Verification items for the finished model (mm, model axes). A direction names the side the tool comes from. Give positions to 0.01 mm unless a question says otherwise; leave off trailing zeros. Loops run counter-clockwise (first coordinate to the right, second up) from the corner with the lowest first, then second, coordinate; pieces in that order, holes last. Notation, with made-up numbers: (6.5, -5.75) - (56.5, -5.75) arc R15 cw to (56.5, 14.25) - close; hole circle Ø8 at (-12.5, 75.25). An arc over 180 degrees is marked (long way). One line per item, written item: value. Start each with the question number.
1. Sectioned sample at B-B (x = -25). Record the cut outline in (y, z).
2. Gauge pin test, flat ends, axial feed: pin 1 (12.5 mm diameter, centred on x = -67, y = 50, fed in from +Z); pin 2 (1 mm diameter, centred on y = 3.5, z = 1.5, fed in from -X); pin 3 (4 mm diameter, centred on x = 52, z = -4.5, fed in from -Y); pin 4 (0.6 mm diameter, centred on x = -48, z = 0.5, fed in from +Y). Record the tip position at first contact, or that the pin passes through.
3. Scan lines: L1, parallel to Y at x = 37.5, z = 1.75; L2, parallel to X at y = 13, z = -14.25; L3, parallel to Z at x = -49, y = 149. Record each from-to range of solid material in increasing order. Write a range as [from, to].
4. Sectioned sample at A-A (z = -4). Record the cut outline in (x, y).
5. Sectioned sample at D-D (x = 78). Record the cut outline in (y, z).
6. Access from +Z, -Z, +X, -X, +Y, -Y to the whole of each face (thin tool, end or side, straight path). Record for faces 1 (the flat face through (94.815, 76, -10)), 2 (the flat face through (0, 17, 2)), 3 (the flat face through (75, 40, 0)), 4 (the flat face through (-77, 40, 0)).
7. Mould release check, pull along Y, two halves, no side actions. Record for faces 5 (the flat face through (1, 0, 1)), 6 (the flat face through (54.815, 74, -10)), 7 (the flat face through (-76, 110, 0)): pulls with the +Y half, pulls with the -Y half, needs draft (parallel to the pull), parting line crosses it, or undercut.
8. Sectioned sample at C-C (y = 67). Record the cut outline in (x, z).
from build123d import *

# Parameters (mm, degrees)
F1_DEPTH = 2
F3_DEPTH = 2
F4_DEPTH = 3
F5_DEPTH = 2
F6_W     = 40
F6_H     = 10
F6_H_2   = 60
F7_DEPTH = 20


with BuildPart() as f1:
    # F0 (on Top) → F1 (new body)
    with BuildSketch(Plane.XY):
        Polygon((-12.130910923, 0), (0, 0), (12.130910923, 0), (12.130910923, 200), (-12.130910923, 200), align=None)
    extrude(amount=F1_DEPTH)

    # F2 (on Top) → F3 (join)
    with BuildSketch(Plane.XY):
        Polygon((-97.5, 0), (0, 0), (97.5, 0), (97.5, 10), (-97.5, 10), align=None)
        Polygon((-97.5, 70), (0, 70), (97.5, 70), (97.5, 80), (-97.8855118155, 80), align=None)
        Polygon((-97.8855118155, 140), (0, 140), (97.5, 140), (97.5, 150), (-97.8855118155, 150), align=None)
    extrude(amount=F3_DEPTH)

    # F2 (on Top) → F4 (join)
    with BuildSketch(Plane.XY):
        Polygon((-97.5, 70), (0, 70), (97.5, 70), (97.5, 80), (-97.8855118155, 80), align=None)
        Polygon((-97.8855118155, 140), (0, 140), (97.5, 140), (97.5, 150), (-97.8855118155, 150), align=None)
    extrude(amount=F4_DEPTH)

    # F2 (on Top) → F5 (join)
    with BuildSketch(Plane.XY):
        Polygon((-97.5, 0), (0, 0), (97.5, 0), (97.5, 10), (-97.5, 10), align=None)
        Polygon((-97.5, 70), (0, 70), (97.5, 70), (97.5, 80), (-97.8855118155, 80), align=None)
        Polygon((-97.8855118155, 140), (0, 140), (97.5, 140), (97.5, 150), (-97.8855118155, 150), align=None)
    extrude(amount=F5_DEPTH)

    # F6 (on face) → F7 (join)
    with BuildSketch(Plane(origin=(0, 0, 0), x_dir=(1, 0, 0), z_dir=(0, 0, -1))):
        Polygon((-57.4945055695, 0), (-97.5, 0), (-97.3342470533, -10), (-57.3287526228, -10), align=None)
        Polygon((-57.3287526228, -10), (-97.3342470533, -10), (-96.3397293732, -70), (-56.3342349427, -70), align=None)
        with Locations((74.8154554615, -5)):
            Rectangle(F6_W, F6_H)
        Polygon((-56.3342349427, -70), (-96.3397293732, -70), (-96.1739764266, -80), (-56.168481996, -80), align=None)
        with Locations((74.8154554615, -40)):
            Rectangle(F6_W, F6_H_2)
        Polygon((-56.168481996, -80), (-96.1739764266, -80), (-95.1794587465, -140), (-55.173964316, -140), align=None)
        with Locations((74.8154554615, -75)):
            Rectangle(F6_W, F6_H)
        Polygon((-55.173964316, -140), (-95.1794587465, -140), (-95.0137057998, -150), (-55.0082113693, -150), align=None)
        with Locations((74.8154554615, -110)):
            Rectangle(F6_W, F6_H_2)
        with Locations((74.8154554615, -145)):
            Rectangle(F6_W, F6_H)
    extrude(amount=F7_DEPTH)


solid = f1.part
Results are:
1. outline: (0, 0) - (10, 0) - (10, 2) - (0, 2) - close; (70, 0) - (80, 0) - (80, 3) - (70, 3) - close; (140, 0) - (150, 0) - (150, 3) - (140, 3) - close
2. pin 1: stops at z = 0
2. pin 2: stops at x = -97.5
2. pin 3: passes through
2. pin 4: stops at y = 150
3. L1: y = [0, 10], [70, 80], [140, 150]
3. L2: x = [-97.28, -57.28], [54.82, 94.82]
3. L3: z = [0, 3]
4. outline: (-97.5, 0) - (-57.49, 0) - (-55.01, 150) - (-95.01, 150) - close; (54.82, 0) - (94.82, 0) - (94.82, 150) - (54.82, 150) - close
5. outline: (0, -20) - (150, -20) - (150, 3) - (140, 3) - (140, 0) - (80, 0) - (80, 3) - (70, 3) - (70, 0) - (10, 0) - (10, 2) - (0, 2) - close
6. face 1: -Z, +X, +Y, -Y
6. face 2: +Z, +X, -X, -Y
6. face 3: +Z, +X
6. face 4: +Z, -X
7. face 5: pulls with the -Y half
7. face 6: needs draft
7. face 7: undercut
8. outline: (-96.39, -20) - (-56.38, -20) - (-56.38, 0) - (-96.39, 0) - close; (-12.13, 0) - (12.13, 0) - (12.13, 2) - (-12.13, 2) - close; (54.82, -20) - (94.82, -20) - (94.82, 0) - (54.82, 0) - close
